from build123d import *

# Parameters (mm, degrees)
BOSS_EXTRUDE1_DEPTH       = 8.2
CUT_EXTRUDE1_DEPTH        = 2.2
SKETCH3_W                 = 6.75
SKETCH3_H                 = 8.2
BOSS_EXTRUDE2_DEPTH       = 2
F_1_5MM_DOWEL_HOLE1_D     = 1.5
F_1_5MM_DOWEL_HOLE1_DEPTH = 3
F_1_5MM_DOWEL_HOLE1_TIP   = 0.450645464
M2X0_4_TAPPED_HOLE1_D     = 1.6
M2X0_4_TAPPED_HOLE1_DEPTH = 3
M2X0_4_TAPPED_HOLE1_TIP   = 0.480688495


with BuildPart() as part:
    # Sketch1 → Boss-Extrude1 (new body)
    with BuildSketch(Plane.XY):
        Polygon((0, 0), (0, 4.787274917), (1.582547561, 6.315523332), (5.75, 2), (6.75, 2), (6.75, 0), align=None)
    extrude(amount=BOSS_EXTRUDE1_DEPTH)

    # Sketch2 → Cut-Extrude1 (cut)
    with BuildSketch(Plane(origin=(3.97472688, 3.838349131, 0), x_dir=(0, 0, -1), z_dir=(0.7193398, 0.69465837, 0))):
        with BuildLine():
            Line((0, 3.443677383), (0, -2.555606029))
            Line((0, -2.555606029), (-6.45, -2.555606029))
            ThreePointArc((-6.45, -2.555606029), (-7.45, -1.555606029), (-6.45, -0.555606029))
            Line((-6.45, -0.555606029), (-6.2, -0.555606029))
            Line((-6.2, -0.555606029), (-6.2, 3.443677383))
            Line((-6.2, 3.443677383), (0, 3.443677383))
        make_face()
    extrude(amount=-CUT_EXTRUDE1_DEPTH, mode=Mode.SUBTRACT)

    # Sketch3 → Boss-Extrude2 (add)
    with BuildSketch(Plane.XZ):
        with Locations((3.375, 4.1)):
            Rectangle(SKETCH3_W, SKETCH3_H)
    extrude(amount=BOSS_EXTRUDE2_DEPTH)

    # Ø1.5mm Dowel Hole1
    with Locations(Plane(origin=(0, -2, 0), x_dir=(-1, 0, 0), z_dir=(0, -1, 0))):
        with Locations((-2, -7.1), (-2, -1.1)):
            Hole(F_1_5MM_DOWEL_HOLE1_D / 2, depth=F_1_5MM_DOWEL_HOLE1_DEPTH)
            with Locations((0, 0, -(F_1_5MM_DOWEL_HOLE1_DEPTH + F_1_5MM_DOWEL_HOLE1_TIP / 2))):  # 118° drill point
                Cone(0, F_1_5MM_DOWEL_HOLE1_D / 2, F_1_5MM_DOWEL_HOLE1_TIP, mode=Mode.SUBTRACT)

    # M2x0.4 Tapped Hole1
    with Locations(Plane(origin=(0, -2, 0), x_dir=(-1, 0, 0), z_dir=(0, -1, 0))):
        with Locations((-2, -4.1)):
            Hole(M2X0_4_TAPPED_HOLE1_D / 2, depth=M2X0_4_TAPPED_HOLE1_DEPTH)
            with Locations((0, 0, -(M2X0_4_TAPPED_HOLE1_DEPTH + M2X0_4_TAPPED_HOLE1_TIP / 2))):  # 118° drill point
                Cone(0, M2X0_4_TAPPED_HOLE1_D / 2, M2X0_4_TAPPED_HOLE1_TIP, mode=Mode.SUBTRACT)


solid = part.part
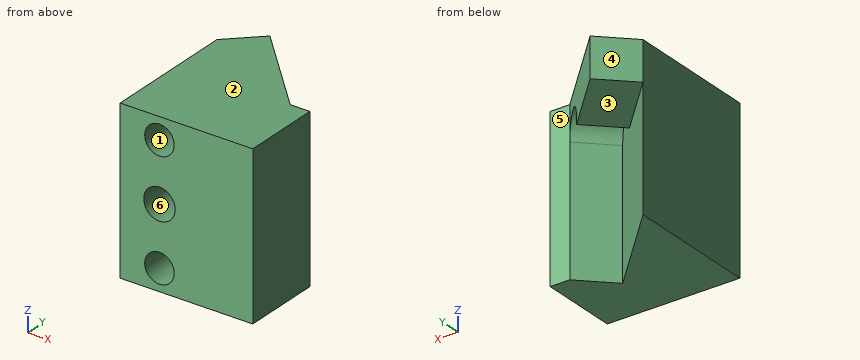
The listing builds one solid part. Answer for the finished solid, in the listing's coordinates (mm). Face numbers are marked on the shaded views. A direction names the side the tool comes from. Give positions to 0.01 mm unless a question says otherwise; leave off trailing zeros. Loops run counter-clockwise (first coordinate to the right, second up) from the corner with the lowest first, then second, coordinate; pieces in that order, holes last. Notation, with made-up numbers: (59.25, 63.5) - (111.25, 63.5) arc R33 cw to (111.25, 100.5) - close; hole circle Ø4 at (-39, 46.5). An arc over 180 degrees is marked (long way). Answer as a JSON object with one key per item and string values.
1. A cutting plane is placed at A-A (z = 6). Write down the section's boundary in (x, y).
Determined:
{"outline": "(0, -2) - (6.75, -2) - (6.75, 2) - (5.75, 2) - (4.17, 0.47) - (0, 4.79) - close"}
2. A cutting plane is placed at C-C (x = 1). Write down the section's boundary in (y, z), then the cut area to 3 significant figures.
Determined:
{"outline": "(-2, 0) - (3.75, 0) - (3.75, 6.2) - (5.75, 6.2) - (5.75, 8.2) - (-2, 8.2) - close", "area": "51.2 mm²"}
3. For a pull along Z with two mould halves and no side action, classify the marked faces 1, 2 and 3 as pulls with the +Z half, pulls with the -Z half, needs draft (parallel to the pull), parting line crosses it, or undercut.
Determined:
{"face 1": "undercut", "face 2": "pulls with the +Z half", "face 3": "pulls with the -Z half"}
4. Flat-ended cylindrical pins translate along their axes: pin 1 Ø3 at (x, z) = (4.5, 1.5) entering from +Y; pin 2 Ø1.3 at (x, z) = (2, 4.1) entering from -Y. Find the tip coordinate at first contact, or state that the pin passes through.
Determined:
{"pin 1": "y = 2", "pin 2": "y = 1.09"}
5. For the marked faces 4, 5 and 6, determine the directions among +Z, -Z, +X, -X, +Y, -Y from which every point of the face is accessible in a straight line to the end or side of a thin tool.
Determined:
{"face 4": "+Z, -Z, -X, +Y", "face 5": "+Z, -Z, +X, +Y", "face 6": "-Y"}
6. A cutting plane is placed at B-B (y = 5.5). Write down the section's boundary in (x, z).
Determined:
{"outline": "(0.74, 6.2) - (2.37, 6.2) - (2.37, 8.2) - (0.74, 8.2) - close"}
7. Find the intervals of material crossed by L1, parallel to Z at x = 2, y = -0.6; L2, parallel to X at y = -0.7, z = 7.1; L3, parallel to Z at x = 1.25, y = 5.5, in increasing order. Write a range as [from, to].
Determined:
{"L1": "[0, 0.35], [1.85, 3.3], [4.9, 6.35], [7.85, 8.2]", "L2": "[0, 1.25], [2.75, 6.75]", "L3": "[6.2, 8.2]"}
